Autodesk Inventor part; units mm, degrees
ref_plane "YZ Plane" through (0, 0, 0) normal (1, 0, 0) x (0, 1, 0)
ref_plane "XZ Plane" through (0, 0, 0) normal (0, 1, 0) x (-1, 0, 0)
ref_plane "XY Plane" through (0, 0, 0) normal (0, 0, 1) x (1, 0, 0)
sketch "Sketch1" plane through (0, 0, 0) normal (0, 0, 1) x (1, 0, 0)
  circle A0 centre (0, 0) radius 11.1125
  dimension "d0" = 22.225
extrude "Extrusion1" add sketch "Sketch1" along normal mid plane 25.4
sketch "Sketch3" plane through (0, 0, -12.7) normal (0, 0, -1) x (-1, 0, 0)
  circle A0 centre (0, 0) radius 11.1125
  circle A1 centre (0, 0) radius 6.35
  dimension "d6" = 12.7
extrude "Extrusion3" cut sketch "Sketch3" against normal blind 15.875
sketch "Sketch5" plane through (0, 0, -12.7) normal (0, 0, -1) x (-1, 0, 0)
  circle A0 centre (0, 0) radius 6.35 construction
hole "Hole2" at (0, 0, -12.7) direction (0, 0, 1) diameter 6.35 end through all
properties part number "AR-013" material "Aluminum 6061"
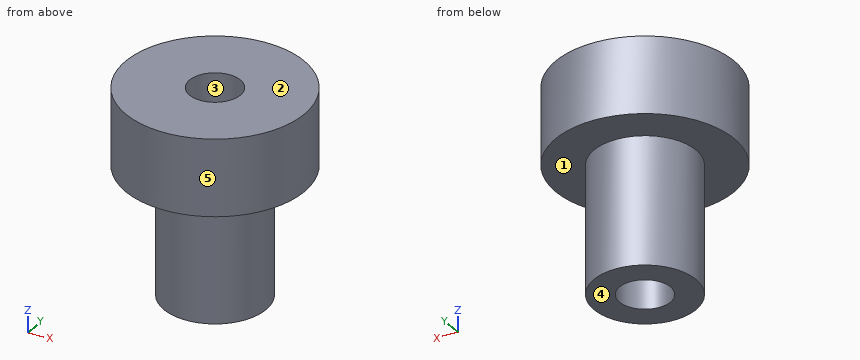
Here's how the part is built. I have some questions about the finished solid (model axes, mm). Face numbers are marked on the shaded views. A direction names the side the tool comes from. Give positions to 0.01 mm unless a question says otherwise; leave off trailing zeros. Write each loop counter-clockwise with the first axis right and the second up, starting at its lowest first coordinate (ties: lowest second). Pieces come first, ordered by that corner, then holes.
(1) Will these pins go through, and if not, where does the flat tip stop? pin 1 (2 mm diameter, centred on x = 7.5, y = -3.5, fed in from -Z) (3 decimals); pin 2 (4 mm diameter, centred on x = 0, y = 0, fed in from -Z) (3 decimals); pin 3 (4 mm diameter, centred on x = 6, z = 1.5, fed in from -Y); pin 4 (6 mm diameter, centred on y = 8.5, z = -7.5, fed in from -X).
Output values:
pin 1: stops at z = 3.175
pin 2: passes through
pin 3: stops at y = -9.97
pin 4: stops at x = -3.17
(2) Imagine slicing it at D-D, the plane y = 4.75. Write out the boundary of the cut face in (x, z) (3 decimals).
Output values:
outline: (-10.046, 3.175) - (-4.214, 3.175) - (-4.214, -12.7) - (4.214, -12.7) - (4.214, 3.175) - (10.046, 3.175) - (10.046, 12.7) - (-10.046, 12.7) - close
(3) On a 3-axis mill with a long thin cutter (end or side, diameter ignored), from which of +Z, -Z, +X, -X, +Y, -Y can I reach the whole of each face in a straight line? I mean the marked faces 1 and 2. Say none if no direction works.
Output values:
face 1: -Z
face 2: +Z, +X, -X, +Y, -Y
(4) Thinking about a two-plate mould opening in X: for the marked faces 3, 4 and 5, which applies, pulls with the +X half, pulls with the -X half, needs draft (parallel to the pull), parting line crosses it, or undercut?
Output values:
face 3: undercut
face 4: needs draft
face 5: parting line crosses it
(5) Imagine slicing it at C-C, the plane z = 2.25. Write out the boundary of the cut face in (x, y) (3 decimals), and give its area (3 significant figures).
Output values:
outline: circle Ø12.7 at (0, 0); hole circle Ø6.35 at (0, 0)
area: 95.0 mm2
(6) If I drill on L1, parallel to Y at x = 0, z = 4 (1 decimal); L2, parallel to Y at x = 0, z = -0.5 (3 decimals); L3, parallel to Z at x = -3.25, y = 7.5 (3 decimals), over which ranges is the centre line in solid material (lowest first)?
Output values:
L1: y = -11.1 to -3.2, 3.2 to 11.1
L2: y = -6.35 to -3.175, 3.175 to 6.35
L3: z = 3.175 to 12.7
